Here's the drawing with two shaded views (mm, measured from the low corner). I have some questions. A direction names the side the tool comes from. Round coordinates to 2 decimals unless told otherwise and drop trailing zeros. Write each loop counter-clockwise with the first axis right and the second up, starting at its lowest first coordinate (ties: lowest second). Pieces come first, ordered by that corner, then holes. Notation, with made-up numbers: M 79.5,-36.5 L 118.5,-36.5 A16 ccw 118.5,-12.5 Z; hole C -18.5,13 d8. An arc over 180 degrees is marked long. Answer as a JSON object with one key per item and string values. Group by question number.
1) Suppose I cut it at B-B, the plane x = 100. Write out the boundary of the cut face in (y, z), and give its area (3 significant figures).
2) On a 3-axis mill with a long thin cutter (end or side, diameter ignored), from which of +Z, -Z, +X, -X, +Y, -Y can I reach the whole of each face in a straight line? I mean the marked faces 1, 2 and 3. Say none if no direction works.
3) Suppose I cut it at A-A, the plane z = 18. Write out the boundary of the cut face in (x, y).
4) Suppose I cut it at C-C, the plane y = 79.5. Write out the boundary of the cut face in (x, z), and give its area (3 significant figures).
5) If we mould it in two halves opening along Z, with no side actions, what happens to the marked faces 4, 5 and 6? For each: +Z half, -Z half, draft (parallel to the pull), parting line (faces both ways), or undercut.
6) Please list where these lines run through material, in increasing order: L1, parallel to Z at x = 100, y = 23; L2, parallel to Z at x = 97, y = 16; L3, parallel to X at y = 23, z = 18. Write a range as [from, to].
7) I'm going to push flat-ended pins straight in: pin 1 Ø12 at (x, y) = (24.5, 79) entering from -Z; pin 2 Ø12 at (y, z) = (31.5, 36) entering from -X; pin 3 Ø5 at (x, z) = (52.5, 56.5) entering from +Y. Where does each tip first touch, or does it pass through?
8) Suppose I cut it at D-D, the plane z = 67.5. Write out the boundary of the cut face in (x, y).
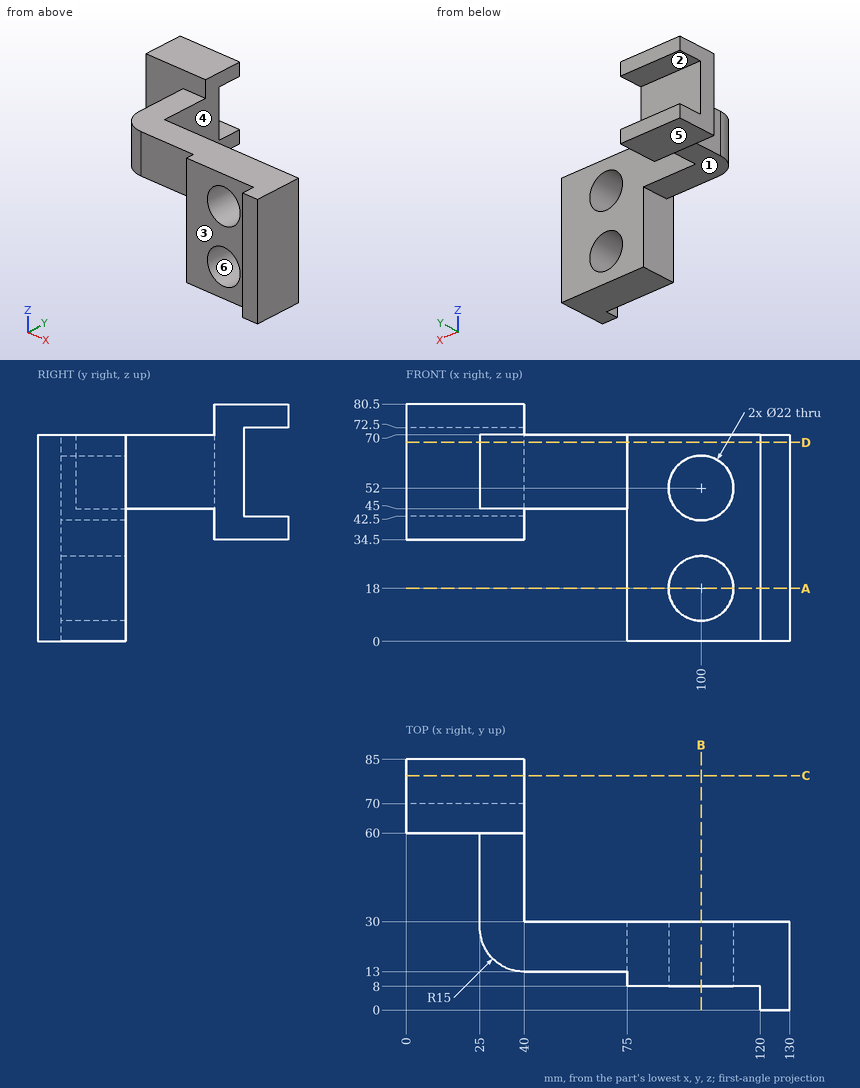
Results:
{
 "1": {"outline": "M 8,0 L 30,0 L 30,7 L 8,7 Z; M 8,29 L 30,29 L 30,41 L 8,41 Z; M 8,63 L 30,63 L 30,70 L 8,70 Z", "area": "572 mm^2"},
 "2": {"face 1": "-Z, -X, -Y", "face 2": "+X, -X, +Y", "face 3": "+Z, -Z, -X, -Y"},
 "3": {"outline": "M 75,8 L 89,8 L 89,30 L 75,30 Z; M 111,8 L 120,8 L 120,0 L 130,0 L 130,30 L 111,30 Z"},
 "4": {"outline": "M 0,34.5 L 40,34.5 L 40,42.5 L 0,42.5 Z; M 0,72.5 L 40,72.5 L 40,80.5 L 0,80.5 Z", "area": "640 mm^2"},
 "5": {"face 4": "draft", "face 5": "-Z half", "face 6": "undercut"},
 "6": {"L1": "[0, 7], [29, 41], [63, 70]", "L2": "[0, 7.42], [28.58, 41.42], [62.58, 70]", "L3": "[75, 89], [111, 130]"},
 "7": {"pin 1": "z = 34.5", "pin 2": "x = 75", "pin 3": "y = 30"},
 "8": {"outline": "M 0,60 L 25,60 L 25,28 A15 ccw 40,13 L 75,13 L 75,8 L 120,8 L 120,0 L 130,0 L 130,30 L 40,30 L 40,70 L 0,70 Z"}
}
